Source: CAD feature listing. Evaluate the final solid. Frame: model axes, mm. A direction names the side the tool comes from. Give positions to 0.01 mm unless a question says otherwise; leave off trailing zeros. Write each loop counter-clockwise with the first axis right and the second up, starting at its lowest first coordinate (ties: lowest second). Pieces come first, ordered by that corner, then holes. Notation, with made-up numbers: (58, -32) -> (71, -32) arc R21 ccw to (71, 4) -> close; hole circle Ø3 at (9, 87.25). An arc over 180 degrees is marked (long way). Write item = value, one per line.
from build123d import *

# Parameters (mm, degrees)
SKETCH1_W           = 10
SKETCH1_H           = 10
BOSS_EXTRUDE1_DEPTH = 10
SKETCH3_R           = 1
CUT_EXTRUDE1_DEPTH  = 1


with BuildPart() as part:
    # Sketch1 → Boss-Extrude1 (new body)
    with BuildSketch(Plane.XY):
        with Locations((5, 5)):
            Rectangle(SKETCH1_W, SKETCH1_H)
    extrude(amount=-BOSS_EXTRUDE1_DEPTH)

    # Sketch3 → Cut-Extrude1 (cut)
    with BuildSketch(Plane(origin=(0, 0, -5), x_dir=(-1, 0, 0), z_dir=(0, 0, -1))):
        with Locations((-8.022028726, 7.600171924)):
            Circle(SKETCH3_R)
    extrude(amount=-CUT_EXTRUDE1_DEPTH, mode=Mode.SUBTRACT)


solid = part.part
1) Draft query along X for faces 3 (the flat face through (5, 5, -10)), 4 (the cylindrical face through (8.816, 6.992, -4.507)), 5 (the flat face through (10, 5, -5)), 6 (the flat face through (0, 5, -5)). Return one class per face: pulls with the +X half, pulls with the -X half, needs draft (parallel to the pull), parting line crosses it, or undercut.
Computed:
face_3 = needs draft
face_4 = undercut
face_5 = pulls with the +X half
face_6 = pulls with the -X half
2) Material intervals for L1, parallel to Z at x = 7.75, y = 7.25, sorted ascending.
Computed:
L1 = -10 to -5, -4 to 0
3) Access query for faces 1 (the flat face through (5, 0, -5)), 2 (the flat face through (8, 8, -4)). Directions: +Z, -Z, +X, -X, +Y, -Y. A direction counts if a zero-diameter tool reaches every point of the face in a straight line with its end or side. Return the directions, or none.
Computed:
face_1 = +Z, -Z, +X, -X, -Y
face_2 = none
4) Cut plane A-A (y = 7). Return the cut outline in (x, z), then the cut area to 3 significant figures.
Computed:
outline = (0, -10) -> (10, -10) -> (10, 0) -> (0, 0) -> close; hole (7.22, -5) -> (8.82, -5) -> (8.82, -4) -> (7.22, -4) -> close
area = 98.4 mm²
5) Cut plane B-B (x = 7.5). Return the cut outline in (y, z).
Computed:
outline = (0, -10) -> (10, -10) -> (10, 0) -> (0, 0) -> close; hole (6.75, -5) -> (8.45, -5) -> (8.45, -4) -> (6.75, -4) -> close
